from build123d import *

# Parameters (mm, degrees)
F0_W     = 20
F0_H     = 20
F1_DEPTH = 20
F2_W     = 13.2
F2_H     = 13.2
F3_DEPTH = 16
F4_R     = 5
F5_R     = 2


with BuildPart() as f1:
    # F0 (on Front) → F1 (new body)
    with BuildSketch(Plane.XZ):
        with Locations((10, 10)):
            Rectangle(F0_W, F0_H)
    extrude(amount=F1_DEPTH)

    # F2 (on face) → F3 (cut)
    with BuildSketch(Plane(origin=(0, 0, 0), x_dir=(-1, 0, 0), z_dir=(0, 1, 0))):
        with Locations((-10, 10)):
            Rectangle(F2_W, F2_H)
    extrude(amount=-F3_DEPTH, mode=Mode.SUBTRACT)

    # F4
    f4_edges = [f1.edges().sort_by_distance(p)[0] for p in [
        (0, -20, 10),
        (10, -20, 0),
        (20, -20, 10),
        (10, -20, 20),
        (20, -10, 20),
        (0, -10, 20),
        (20, -10, 0),
        (0, -10, 0),
    ]]
    fillet(f4_edges, radius=F4_R)

    # F5
    f5_edges = [f1.edges().sort_by_distance(p)[0] for p in [
        (18.535534, 0, 1.464466),
        (20, 0, 10),
        (18.535534, 0, 18.535534),
        (10, 0, 20),
        (1.464466, 0, 18.535534),
        (0, 0, 10),
        (1.464466, 0, 1.464466),
        (10, 0, 0),
    ]]
    fillet(f5_edges, radius=F5_R)


solid = f1.part
Design review of the part built by this model. Coordinates are the model's own, in mm. A direction names the side the tool comes from. Round coordinates to 2 decimals unless told otherwise and drop trailing zeros. Loops run counter-clockwise (first coordinate to the right, second up) from the corner with the lowest first, then second, coordinate; pieces in that order, holes last. Notation, with made-up numbers: (82, 30.5) -> (128, 30.5) arc R7 ccw to (128, 39.5) -> close; hole circle Ø4 at (29, -24.75). An arc over 180 degrees is marked (long way). Use one line per item in the form item = value. Start each with the question number.
Q1. Machinability: for faces 4 (the face through (9.93, -0.57, 19.4)), 5 (the face through (10, -8, 3.4)), which of the approach directions +Z, -Z, +X, -X, +Y, -Y give a long, thin tool a straight path to every point of the face, cutting with its end or side? Answer none if there is none.
Q2. We need section B-B on z = 11.75. Give the boundary of the cut face in (x, y).
Q3. Draft analysis for pull direction Z (two halves, no side actions). For faces 1 (the face through (1, -9, 2)), 2 (the face through (16.6, -8, 10)), 3 (the face through (0.6, -0.57, 9.93)), state which applies: +Z half, -Z half, draft (parallel to the pull), parting line (faces both ways), or undercut.
Q4. Wall thickness on line 1 along X through (y, z) = (-6, 9.5); line 2 along Y through (x, z) = (6.5, 6.25): over which ranges is each line inside the solid? List them lowest first. Write a range as [from, to].
Q5. We need section C-C on x = 10.5. Give the boundary of the cut face in (y, z), then the cut area to 3 significant figures.
Q6. We need section A-A on y = -11.5. Give the boundary of the cut face in (x, z).
Calculated:
q1.face_4 = +Z, +X, -X, +Y
q1.face_5 = +Y
q2.outline = (0, -15) arc R5 ccw to (5, -20) -> (15, -20) arc R5 ccw to (20, -15) -> (20, -2) arc R2 ccw to (18, 0) -> (16.6, 0) -> (16.6, -16) -> (3.4, -16) -> (3.4, 0) -> (2, 0) arc R2 ccw to (0, -2) -> close
q3.face_1 = -Z half
q3.face_2 = undercut
q3.face_3 = draft
q4.line_1 = [0, 3.4], [16.6, 20]
q4.line_2 = [-20, -16]
q5.outline = (-20, 5) arc R5 ccw to (-15, 0) -> (-2, 0) arc R2 ccw to (0, 2) -> (0, 3.4) -> (-16, 3.4) -> (-16, 16.6) -> (0, 16.6) -> (0, 18) arc R2 ccw to (-2, 20) -> (-15, 20) arc R5 ccw to (-20, 15) -> close
q5.area = 176 mm²
q6.outline = (0, 5) arc R5 ccw to (5, 0) -> (15, 0) arc R5 ccw to (20, 5) -> (20, 15) arc R5 ccw to (15, 20) -> (5, 20) arc R5 ccw to (0, 15) -> close; hole (3.4, 3.4) -> (16.6, 3.4) -> (16.6, 16.6) -> (3.4, 16.6) -> close
